Read the model definition and answer for the solid it produces. Units are mm, in the model's axes. A direction names the side the tool comes from. Give positions to 0.01 mm unless a question says otherwise; leave off trailing zeros. Loops run counter-clockwise (first coordinate to the right, second up) from the corner with the lowest first, then second, coordinate; pieces in that order, holes last.
(1) Find section B-B, the plane z = 0. Write down the section's boundary in (x, y).
(2) Find section C-C, the plane x = 100. Write down the section's boundary in (y, z).
(3) Find section D-D, the plane y = -2.5. State how many separate pieces and enclosed holes the cut face has, then the cut area to 3 significant figures.
(4) Find section A-A, the plane x = 45. Write down the section's boundary in (y, z), then the cut area to 3 significant figures.
(5) Each of these flat-tipped pins is pushed along its axis until it touches: P1, Ø12, axis at y = 5, z = -4, coming from the -X side; P2, Ø6, axis at x = 45, y = -5, coming from the -Z side; P3, Ø7.5, axis at x = 98, z = 1.5, coming from the +Y side; P4, Ø5, axis at x = 60, y = -12, coming from the +Z side. Where does it stop, or does it pass through?
(6) Straight lines are drawn through the part: probe 1 along Z at (x, y) = (100, -0.5); probe 2 along X at (y, z) = (-4, 9.5); probe 3 along Z at (x, y) = (45, -4). For each, find the intervals that lie inside material, in ascending order.
(7) Which of the six approach directions +Z, -Z, +X, -X, +Y, -Y give full straight-line access (tool end or side, diameter ignored) to faces 1 (the face through (48, -12, 6)), 2 (the face through (51, 12, -3)), 3 (the face through (73.209, -1.396, -6.288)), 4 (the face through (104.496, 0.367, -0.198)), 5 (the face through (38.655, -0.168, -1.409))?
```python
from build123d import *
from build123d.topology import SkipClean

# Parameters (mm, degrees)
SKETCH2_R                  = 14.892385846
CUT_EXTRUDE1_DEPTH         = 10
M10X1_0_TAPPED_HOLE1_D     = 9
M10X1_0_TAPPED_HOLE1_DEPTH = 19
CUT_EXTRUDE2_DEPTH         = 116.190060335
CUT_EXTRUDE2_DEPTH_BACK    = 116.190060335
SKETCH5_W                  = 33.852396008
SKETCH5_H                  = 3.402803332
SKETCH5_H_2                = 3.72687984
CUT_EXTRUDE3_DEPTH         = 118.612711898
CUT_EXTRUDE3_DEPTH_BACK    = 118.612711898
SKETCH6_R                  = 6.5
SKETCH7_R                  = 1.5
CUT_EXTRUDE5_DEPTH         = 12


with BuildPart() as part:
    # Sketch1 → Revolve1 (revolve)
    with SkipClean():  # the faces are left unmerged after this step: merging them gives an invalid solid
        with BuildSketch(Plane.XY):
            with BuildLine():
                ThreePointArc((14.361406616, 10), (-5.240485866, 16.696925103), (-17.5, 0))
                Line((-17.5, 0), (17.5, 0))
                ThreePointArc((17.5, 0), (16.696925103, 5.240485866), (14.361406616, 10))
            make_face()
            with BuildLine():
                Line((17.5, 0), (-17.5, 0))
                ThreePointArc((-17.5, 0), (0, -17.5), (17.5, 0))
            make_face()
            with BuildLine():
                ThreePointArc((14.361406616, 10), (16.696925103, 5.240485866), (17.5, 0))
                Line((17.5, 0), (30, 0))
                ThreePointArc((30, 0), (30.745975783, 4.671487304), (32.909705817, 8.87833242))
                Line((32.909705817, 8.87833242), (14.361406616, 10))
            make_face()
            with BuildLine():
                ThreePointArc((58.072071664, 7.356693714), (45.905437929, 14.9726478), (32.909705817, 8.87833242))
                Line((32.909705817, 8.87833242), (58.072071664, 7.356693714))
            make_face()
            with BuildLine():
                ThreePointArc((32.909705817, 8.87833242), (30.745975783, 4.671487304), (30, 0))
                Line((30, 0), (60, 0))
                ThreePointArc((60, 0), (59.510015075, 3.802559995), (58.072071664, 7.356693714))
                Line((58.072071664, 7.356693714), (32.909705817, 8.87833242))
            make_face()
            with BuildLine():
                ThreePointArc((58.072071664, 7.356693714), (59.510015075, 3.802559995), (60, 0))
                Line((60, 0), (87.5, 0))
                ThreePointArc((87.5, 0), (87.822928267, 2.822928267), (88.77502784, 5.5))
                Line((88.77502784, 5.5), (58.072071664, 7.356693714))
            make_face()
            with BuildLine():
                ThreePointArc((88.77502784, 5.5), (87.822928267, 2.822928267), (87.5, 0))
                Line((87.5, 0), (112.5, 0))
                ThreePointArc((112.5, 0), (102.822928267, 12.177071733), (88.77502784, 5.5))
            make_face()
            with BuildLine():
                Line((112.5, 0), (87.5, 0))
                ThreePointArc((87.5, 0), (100, -12.5), (112.5, 0))
            make_face()
        revolve(axis=Axis((-17.5, 0, 0), (1, 0, 0)))
    add(part.part.scale(1), mode=Mode.REPLACE)  # the faces are merged on a copy

    # Sketch2 → Cut-Extrude1 (cut)
    with BuildSketch(Plane(origin=(0, 10, 0), x_dir=(1, 0, 0), z_dir=(0, 1, 0))):
        with Locations((100, 0)):
            Circle(SKETCH2_R)
    extrude(amount=CUT_EXTRUDE1_DEPTH, mode=Mode.SUBTRACT)

    # M10x1.0 Tapped Hole1
    with Locations(Plane(origin=(0, 10, 0), x_dir=(1, 0, 0), z_dir=(0, 1, 0))):
        with Locations((100, 0)):
            Hole(M10X1_0_TAPPED_HOLE1_D / 2, depth=M10X1_0_TAPPED_HOLE1_DEPTH)

    # Sketch5 → Cut-Extrude2 (cut, two sides: drawn at the far end of the back side and taken through both)
    with BuildSketch(Plane.XY.offset(-CUT_EXTRUDE2_DEPTH_BACK)):
        with Locations((45.092145357, 13.701401666)):
            Rectangle(SKETCH5_W, SKETCH5_H)
        with Locations((45.092145357, -13.86343992)):
            Rectangle(SKETCH5_W, SKETCH5_H_2)
    extrude(amount=CUT_EXTRUDE2_DEPTH + CUT_EXTRUDE2_DEPTH_BACK, mode=Mode.SUBTRACT)

    # Sketch6 → Cut-Extrude3 (cut, two sides: drawn at the far end of the back side and taken through both)
    with BuildSketch(Plane(origin=(0, 12, 0), x_dir=(1, 0, 0), z_dir=(0, 1, 0)).offset(-CUT_EXTRUDE3_DEPTH_BACK)):
        with Locations(Location((45, 0, 0), (0, 0, 270))):
            Circle(SKETCH6_R)
    extrude(amount=CUT_EXTRUDE3_DEPTH + CUT_EXTRUDE3_DEPTH_BACK, mode=Mode.SUBTRACT)

    # Sketch7 → Cut-Extrude5 (cut)
    with BuildSketch(Plane(origin=(0, 12, 0), x_dir=(1, 0, 0), z_dir=(0, 1, 0))):
        with Locations((38.103493706, 0)):
            Circle(SKETCH7_R)
    extrude(amount=-CUT_EXTRUDE5_DEPTH, mode=Mode.SUBTRACT)


solid = part.part
```
Entries:
1. outline: (14.36, -10) - (32.91, -8.88) arc R15 ccw to (36, -12) - (38.5, -12) - (38.5, 0) - (36.6, 0) - (36.6, 12) - (36, 12) arc R15 ccw to (32.91, 8.88) - (14.36, 10) arc R17.5 ccw (long way) to start; (51.5, -12) - (54, -12) arc R15 ccw to (58.07, -7.36) - (88.78, -5.5) arc R12.5 ccw (long way) to (107.5, 10) - (104.5, 10) - (104.5, -9) - (95.5, -9) - (95.5, 10) - (92.5, 10) arc R12.5 ccw to (88.78, 5.5) - (58.07, 7.36) arc R15 ccw to (54, 12) - (51.5, 12) - close
2. outline: (-9, -4.5) - (-9, 4.5) - (10, 4.5) - (10, 7.5) arc R12.5 ccw (long way) to (10, -7.5) - (10, -4.5) - close
3. separate pieces: 1
3. enclosed holes: 2
3. area: 2,510 mm2
4. outline: (-12, -9) arc R15 ccw to (12, -9) - (12, -6.5) - (-12, -6.5) - close; (-12, 6.5) - (12, 6.5) - (12, 9) arc R15 ccw to (-12, 9) - close
4. area: 321 mm2
5. P1: stops at x = -17.5
5. P2: stops at z = -14.87
5. P3: stops at y = 10
5. P4: passes through
6. probe 1: z = -12.49 to -4.5, 4.5 to 12.49
6. probe 2: x = -14.14 to 14.14, 34.1 to 55.9, 92.93 to 107.07
6. probe 3: z = -14.46 to -6.5, 6.5 to 14.46
7. face 1: +Z, -Z, -Y
7. face 2: +Z, -Z, +X, +Y
7. face 3: none
7. face 4: +Y
7. face 5: +Y, -Y
